Geometry check sheet. Reference: the model listing, model coordinates, mm. A direction names the side the tool comes from. Coordinates: 2 decimals unless noted, no trailing zeros. Write each loop counter-clockwise with the first axis right and the second up, starting at its lowest first coordinate (ties: lowest second). Pieces come first, ordered by that corner, then holes. Notation, with made-up numbers: (71.5, 65) -> (77.5, 65) arc R11 ccw to (77.5, 74) -> close; hole circle Ø5 at (-20.5, 57). An arc over 180 degrees is marked (long way). One line per question, with ' | ' between items.
from build123d import *

# Parameters (mm, degrees)
BOSS_EXTRUDE1_DEPTH = 6
BOSS_EXTRUDE2_DEPTH = 6
SKETCH3_R           = 2
CUT_EXTRUDE1_DEPTH  = 6
FILLET1_R           = 1


with BuildPart() as part:
    # Sketch1 → Boss-Extrude1 (new body)
    with BuildSketch(Plane(origin=(0, 0, 0), x_dir=(1, 0, 0), z_dir=(0, 1, 0))):
        with BuildLine():
            Line((5, 0), (7, 0))
            ThreePointArc((7, 0), (0, 7), (-7, 0))
            Line((-7, 0), (-5, 0))
            ThreePointArc((-5, 0), (0, 5), (5, 0))
        make_face()
    extrude(amount=BOSS_EXTRUDE1_DEPTH)

    # Sketch2 → Boss-Extrude2 (add)
    with BuildSketch(Plane(origin=(0, 6, 0), x_dir=(1, 0, 0), z_dir=(0, 1, 0))):
        Polygon((7, 0), (13, 0), (13, 2), (6.708203932, 2), align=None)
        Polygon((-6.708203932, 2), (-7, 0), (-13, 0), (-13, 2), align=None)
    extrude(amount=-BOSS_EXTRUDE2_DEPTH)

    # Sketch3 → Cut-Extrude1 (cut)
    with BuildSketch(Plane(origin=(0, 0, -2), x_dir=(-1, 0, 0), z_dir=(0, 0, -1))):
        with Locations((-9.5, 3)):
            Circle(SKETCH3_R)
        with Locations((9.5, 3)):
            Circle(SKETCH3_R)
    extrude(amount=-CUT_EXTRUDE1_DEPTH, mode=Mode.SUBTRACT)

    # Fillet1
    fillet1_edges = [part.edges().sort_by_distance(p)[0] for p in [
        (13, 6, -1),
        (13, 0, -1),
        (-13, 6, -1),
        (-13, 0, -1),
        (-5, 3, 0),
        (5, 3, 0),
    ]]
    fillet(fillet1_edges, radius=FILLET1_R)


solid = part.part
1. Mould release check, pull along X, two halves, no side actions. Record for faces 1 (the face through (11.3, 4.4, -2)), 2 (the face through (5.28, 3.04, -0.23)), 3 (the face through (-12.699, 5.715, -1.014)): released by +X, released by -X, zero draft, split by the parting line, or undercut.
Worked answers:
face 1: zero draft | face 2: undercut | face 3: released by -X
2. Cross-section at B-B on x = -9.5. Record the boundary of the cut face in (y, z), and give its area (3 significant figures).
Worked answers:
outline: (0, -2) -> (1, -2) -> (1, 0) -> (0, 0) -> close; (5, -2) -> (6, -2) -> (6, 0) -> (5, 0) -> close | area: 4.00 mm²
3. Tool access check on faces 4 (the face through (12.715, 0.301, -1.014)), 5 (the face through (-11.3, 4.4, -2)), 6 (the face through (-5.263, 3.042, -0.243)). Record the directions out of +Z, -Z, +X, -X, +Y, -Y that give a thin tool (end or side, any length) a straight path to the whole face; none if there is none.
Worked answers:
face 4: +Z, -Z, +X, -Y | face 5: -Z, -X, +Y, -Y | face 6: +Z, +Y, -Y
4. Cross-section at D-D on y = 5.6. Record the boundary of the cut face in (x, z), and give its area (3 significant figures).
Worked answers:
outline: (-12.8, -2) -> (-6.71, -2) arc R7 ccw to (6.71, -2) -> (12.8, -2) -> (12.8, 0) -> (5.92, 0) arc R1 ccw to (4.93, -0.83) arc R5 cw to (-4.93, -0.83) arc R1 ccw to (-5.92, 0) -> (-12.8, 0) -> close | area: 61.0 mm²
5. Cross-section at A-A on y = 3. Record the boundary of the cut face in (x, z).
Worked answers:
outline: (-13, -2) -> (-11.5, -2) -> (-11.5, 0) -> (-13, 0) -> close; (-7.5, -2) -> (-6.71, -2) arc R7 ccw to (6.71, -2) -> (7.5, -2) -> (7.5, 0) -> (5.92, 0) arc R1 ccw to (4.93, -0.83) arc R5 cw to (-4.93, -0.83) arc R1 ccw to (-5.92, 0) -> (-7.5, 0) -> close; (11.5, -2) -> (13, -2) -> (13, 0) -> (11.5, 0) -> close
6. Go/stop test with flat-tipped pins: P1, Ø1, axis at y = 5, z = -5, coming from the -X side; P2, Ø3, axis at x = 9, y = 1.5, coming from the -Z side. Record where each tip stops, or that it passes through.
Worked answers:
P1: x = -5.36 | P2: z = -2
7. Material ranges on line 1 (Y direction, x = -9.5, z = -0.45); line 2 (X direction, y = 1.35, z = -4.25); line 3 (X direction, y = 2.4, z = -1.25), recorded low to high. Write a range as from..to.
Worked answers:
line 1: 0..1, 5..6 | line 2: -5.56..-2.63, 2.63..5.56 | line 3: -13..-11.41, -7.59..-4.84, 4.84..7.59, 11.41..13
8. Cross-section at C-C on z = -2.5. Record the boundary of the cut face in (x, y).
Worked answers:
outline: (-6.54, 0) -> (-4.33, 0) -> (-4.33, 6) -> (-6.54, 6) -> close; (4.33, 0) -> (6.54, 0) -> (6.54, 6) -> (4.33, 6) -> close
